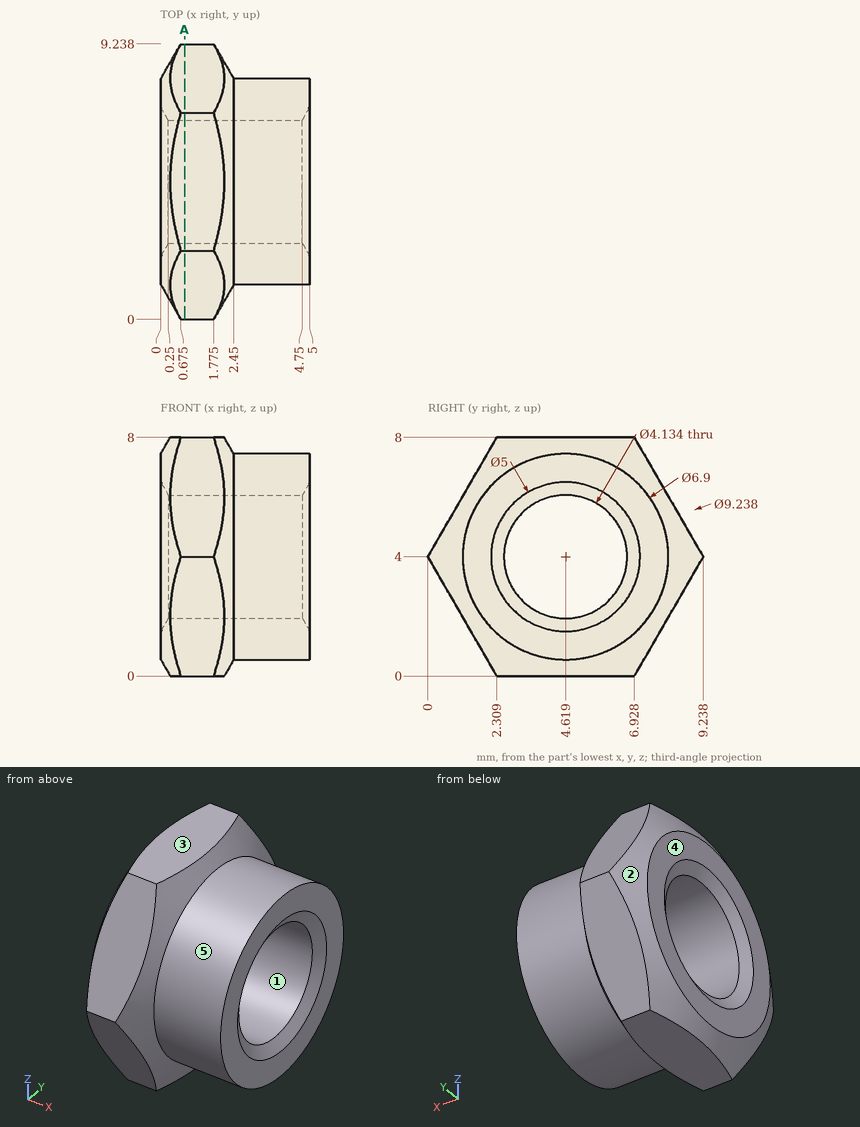
Verification items for this drawing (mm, ordinates from the low corner). A direction names the side the tool comes from. Coordinates: 2 decimals unless noted, no trailing zeros. Order: outer loops, then holes, each group sorted by start corner. A loop starts at its lowest first (then second) coordinate and runs counter-clockwise, first axis right, second up. Notation, with made-up numbers: (-10, 68.5) -> (35, 68.5) arc R23 ccw to (35, 89.5) -> close; hole circle Ø8 at (31, -30). An arc over 180 degrees is marked (long way). Answer as CSV lines item,"result". Start each with the question number.
1) Gauge pin test, flat end, axial feed: pin 1 Ø2 at (x, y) = (4, 8) entering from +Z (1 decimal). Record the tip position at first contact, or that the pin passes through.
2) Set-up check for the marked faces 4 and 5: record each of +Z, -Z, +X, -X, +Y, -Y from which the full face is reachable in a straight line by a thin tool's end or side.
3) Release check for a two-part mould opening along Z. For the marked faces 1, 2 and 3 record: released by +Z, released by -Z, zero draft, split by the parting line, or undercut.
4) Cross-section at A-A, the plane x = 0.8. Record the boundary of the cut face in (y, z).
5) Material ranges on L1, parallel to Y at x = 3.15, z = 4 (1 decimal); L2, parallel to Z at x = 0.55, y = 4.25; L3, parallel to Z at x = 3.4, y = 6.25, recorded low to high. Write a range as [from, to].
Conclusion:
1,pin 1,"stops at z = 6.5"
2,face 4,"+Z, -Z, -X, +Y, -Y"
2,face 5,"+X"
3,face 1,"undercut"
3,face 2,"split by the parting line"
3,face 3,"released by +Z"
4,outline,"(0, 4) -> (2.31, 0) -> (6.93, 0) -> (9.24, 4) -> (6.93, 8) -> (2.31, 8) -> close; hole circle Ø4.13 at (4.62, 4)"
5,L1,"y = [1.2, 2.6], [6.7, 8.1]"
5,L2,"z = [0, 1.97], [6.03, 8]"
5,L3,"z = [0.96, 2.73], [5.27, 7.04]"
